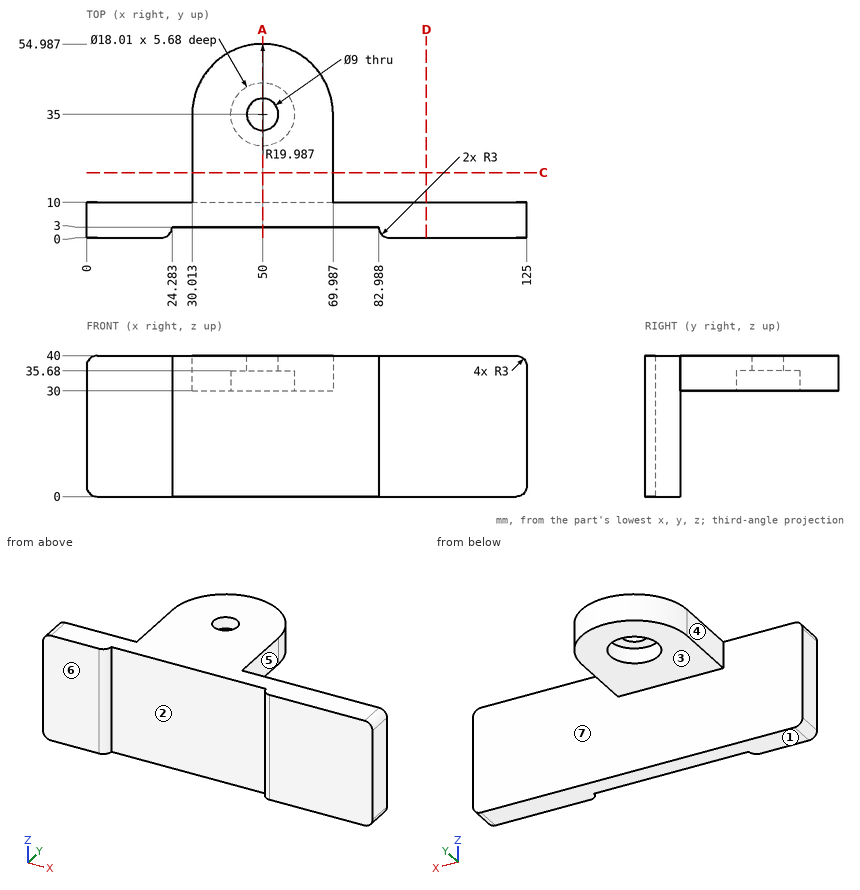
Could you check a few things on this drawing? It's one solid part, dimensions in mm from its lowest x, y, z. A direction names the side the tool comes from. Coordinates: 2 decimals unless noted, no trailing zeros. Write each loop counter-clockwise with the first axis right and the second up, starting at its lowest first coordinate (ties: lowest second). Pieces come first, ordered by that corner, then holes. Notation, with made-up numbers: M 50,24 L 101,24 A25 cw 101,47 Z; hole C 2,76.25 d3. An arc over 180 degrees is marked long. One line per question, with ' | ' between items.
1) I need wall thicknesses on probe 1 along Y at (x, z) = (50, 31) (1 decimal); probe 2 along Z at (x, y) = (66.5, 11); probe 3 along Z at (x, y) = (42.5, 39). Which ranges of each line are inside material? Lowest first, please. Write a range as [from, to].
Checks:
probe 1: [3, 26], [44, 55] | probe 2: [30, 40] | probe 3: [35.68, 40]
2) Imagine slicing it at C-C, the plane y = 18.5. Write out the boundary of the cut face in (x, z).
Checks:
outline: M 30.01,30 L 69.99,30 L 69.99,40 L 30.01,40 Z
3) Imagine slicing it at A-A, the plane x = 50. Write out the boundary of the cut face in (y, z) (1 decimal).
Checks:
outline: M 3,0 L 10,0 L 10,30 L 26,30 L 26,35.7 L 30.5,35.7 L 30.5,40 L 3,40 Z; M 39.5,35.7 L 44,35.7 L 44,30 L 55,30 L 55,40 L 39.5,40 Z
4) For the marked faces 1, 2, 3 and 4, which set-ups out of +Z, -Z, +X, -X, +Y, -Y let a thin tool reach every point of the face, with its end or its side?
Checks:
face 1: -Z, +X, -X, +Y, -Y | face 2: +Z, -Z, -Y | face 3: -Z, +X, -X, +Y | face 4: +Z, -Z, -X, +Y
5) Imagine slicing it at D-D, the plane x = 96.5. Write out the boundary of the cut face in (y, z).
Checks:
outline: M 0,0 L 10,0 L 10,40 L 0,40 Z
6) If we mould it in two halves opening along Y, with no side actions, what happens to the marked faces 5, 6 and 7? For each: released by +Y, released by -Y, zero draft, split by the parting line, or undercut.
Checks:
face 5: zero draft | face 6: released by -Y | face 7: released by +Y
7) For pin 1 Ø16 at (x, y) = (50, 35) entering from -Z; pin 2 Ø1.5 at (x, z) = (50.5, 14) entering from -Y; pin 3 Ø12 at (x, y) = (58.5, 26) entering from -Z; pin 4 Ø4 at (x, y) = (72, 38) entering from +Z, each with a flat end and sliding along its axis, tell me the tip position at first contact or that it passes through.
Checks:
pin 1: z = 35.68 | pin 2: y = 3 | pin 3: z = 30 | pin 4: through
